from build123d import *

# Parameters (mm, degrees)
SKETCH3_W    = 1
SKETCH3_H    = 1
SOFT_EDGES_R = 0.1


with BuildPart() as part:
    # rubber_band: sweep along a path in Sketch2
    with BuildLine(Plane.XY) as rubber_band_path:
        Line((0, 4.5), (86.8, 4.5))
        ThreePointArc((86.8, 4.5), (91.3, 0), (86.8, -4.5))
        Line((86.8, -4.5), (0, -4.5))
        ThreePointArc((0, -4.5), (-4.5, 0), (0, 4.5))
    # Sketch3 → rubber_band (sweep)
    with BuildSketch(Plane(origin=(0, 0, 0), x_dir=(0, 0, -1), z_dir=(1, 0, 0))):
        with Locations((0, 4.5)):
            Rectangle(SKETCH3_W, SKETCH3_H)
    sweep(path=rubber_band_path.line)

    # soft_edges
    soft_edges_edges = [part.edges().sort_by_distance(p)[0] for p in [
        (-5, 0, 0.5),
        (-4, 0, 0.5),
        (-4, 0, -0.5),
        (-5, 0, -0.5),
        (43.4, -5, 0.5),
        (43.4, -4, 0.5),
        (43.4, -4, -0.5),
        (43.4, -5, -0.5),
        (91.8, 0, 0.5),
        (90.8, 0, 0.5),
        (90.8, 0, -0.5),
        (91.8, 0, -0.5),
        (43.4, 5, 0.5),
        (43.4, 4, 0.5),
        (43.4, 4, -0.5),
        (43.4, 5, -0.5),
    ]]
    fillet(soft_edges_edges, radius=SOFT_EDGES_R)


solid = part.part
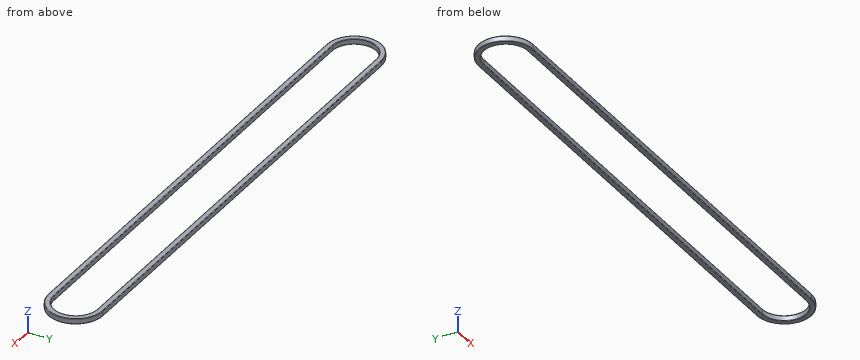
Design review of the part built by this model. Coordinates are the model's own, in mm. Round coordinates to 2 decimals unless told otherwise and drop trailing zeros. Write each loop counter-clockwise with the first axis right and the second up, starting at its lowest first coordinate (ties: lowest second). Pieces come first, ordered by that corner, then holes. Notation, with made-up numbers: M 21.5,71.25 L 66.5,71.25 A22 ccw 66.5,99.25 Z; hole C -8,-3 d1. An arc over 180 degrees is marked long. One line per item, written item: value. Start each with the question number.
1. Take a section at C-C on z = -0.25. State the section outline as (x, y) points.
2. Take a section at B-B on x = 73. State the section outline as (y, z) points.
3. Take a section at A-A on y = 0. State the section outline as (x, z) points, then the cut area to 3 significant figures.
4. To check wall thickness, follow probe 1 along Y at (x, z) = (8, -0.35); probe 2 along X at (y, z) = (-0.25, 0.4); probe 3 along X at (y, z) = (-0.75, 0.15). State the ranges of each line that lie inside material, in increasing order. Write a range as from..to.
Computed:
1. outline: M 0,-5 L 86.8,-5 A5 ccw 86.8,5 L 0,5 A5 ccw Z; hole M 0,-4 L 86.8,-4 A4 ccw 86.8,4 L 0,4 A4 ccw Z
2. outline: M -5,-0.4 A0.1 ccw -4.9,-0.5 L -4.1,-0.5 A0.1 ccw -4,-0.4 L -4,0.4 A0.1 ccw -4.1,0.5 L -4.9,0.5 A0.1 ccw -5,0.4 Z; M 4,-0.4 A0.1 ccw 4.1,-0.5 L 4.9,-0.5 A0.1 ccw 5,-0.4 L 5,0.4 A0.1 ccw 4.9,0.5 L 4.1,0.5 A0.1 ccw 4,0.4 Z
3. outline: M -5,-0.4 A0.1 ccw -4.9,-0.5 L -4.1,-0.5 A0.1 ccw -4,-0.4 L -4,0.4 A0.1 ccw -4.1,0.5 L -4.9,0.5 A0.1 ccw -5,0.4 Z; M 90.8,-0.4 A0.1 ccw 90.9,-0.5 L 91.7,-0.5 A0.1 ccw 91.8,-0.4 L 91.8,0.4 A0.1 ccw 91.7,0.5 L 90.9,0.5 A0.1 ccw 90.8,0.4 Z
3. area: 1.98 mm²
4. probe 1: y = -5..-4, 4..5
4. probe 2: x = -4.99..-3.99, 90.79..91.79
4. probe 3: x = -4.94..-3.93, 90.73..91.74
